Here's how the part is built. I have some questions about the finished solid (model axes, mm). A direction names the side the tool comes from. Give positions to 0.01 mm unless a question says otherwise; leave off trailing zeros. Order: outer loops, then holes, each group sorted by start corner. A loop starts at its lowest first (then second) coordinate and runs counter-clockwise, first axis right, second up.
Autodesk Inventor part; units mm, degrees
ref_plane "YZ Plane" through (0, 0, 0) normal (1, 0, 0) x (0, 1, 0)
ref_plane "XZ Plane" through (0, 0, 0) normal (0, 1, 0) x (-1, 0, 0)
ref_plane "XY Plane" through (0, 0, 0) normal (0, 0, 1) x (1, 0, 0)
sketch "Sketch1" plane through (0, 0, 0) normal (0, 1, 0) x (-1, 0, 0)
  line L0 (90, 60) -> (-90, 60)
  line L1 (-90, 60) -> (-90, -60)
  line L2 (-90, -60) -> (90, -60)
  line L3 (90, -60) -> (90, 60)
  line L4 (90, 60) -> (-90, -60) construction
  line L5 (-90, 60) -> (90, -60) construction
  point P0 (0, 0)
  dimension "d0" = 180
  dimension "d1" = 120
extrude "Extrusion1" add sketch "Sketch1" along normal blind 15
fillet "Face Fillet1" radius 5 1 edges at (90, 7.5, 60)
fillet "Face Fillet2" radius 5 1 edges at (90, 7.5, -60)
fillet "Face Fillet3" radius 5 1 edges at (-90, 7.5, -60)
fillet "Face Fillet4" radius 5 1 edges at (-90, 7.5, 60)
sketch "Sketch2" plane through (0, 15, 0) normal (0, 1, 0) x (1, 0, 0)
  circle A0 centre (0, 0) radius 50
  dimension "d8" = 100
extrude "Extrusion2" add sketch "Sketch2" along normal blind 10
sketch "Sketch3" plane through (0, 25, 0) normal (0, 1, 0) x (1, 0, 0)
  circle A0 centre (0, 0) radius 35
  dimension "d11" = 70
extrude "Extrusion3" add sketch "Sketch3" along normal blind 10
properties part number "base_of weel"
Q1. I need wall thicknesses on L1, parallel to Y at x = 68, z = 5.5; L2, parallel to Y at x = -35, z = 30; L3, parallel to Z at x = 4, y = 29.5. Which ranges of each line are inside material? Lowest first, please.
Filled sheet:
L1: y = 0 to 15
L2: y = 0 to 25
L3: z = -34.77 to 34.77
Q2. If we section it at C-C on y = 31: List the corners of the cut face in (x, z) for me, plus the area to 3 significant figures.
Filled sheet:
outline: circle Ø70 at (0, 0)
area: 3,850 mm2
Q3. If we section it at B-B on z = 0: List the corners of the cut face in (x, y) for me, plus the area to 3 significant figures.
Filled sheet:
outline: (-90, 0) - (90, 0) - (90, 15) - (50, 15) - (50, 25) - (35, 25) - (35, 35) - (-35, 35) - (-35, 25) - (-50, 25) - (-50, 15) - (-90, 15) - close
area: 4,400 mm2
Q4. I'm going to push flat-ended pins straight in: P1, Ø3, axis at x = -54, z = -14, coming from the +Y side; P2, Ø2, axis at y = 24.5, z = 16, coming from the -X side; P3, Ø2, axis at x = 38, z = 14, coming from the +Y side. Where does each tip first touch, or does it pass through?
Filled sheet:
P1: stops at y = 15
P2: stops at x = -47.7
P3: stops at y = 25
Q5. If we section it at A-A on x = 0: List the corners of the cut face in (y, z) for me, plus the area to 3 significant figures.
Filled sheet:
outline: (0, -60) - (15, -60) - (15, -50) - (25, -50) - (25, -35) - (35, -35) - (35, 35) - (25, 35) - (25, 50) - (15, 50) - (15, 60) - (0, 60) - close
area: 3,500 mm2
Q6. If we section it at D-D on x = -65.5: List the corners of the cut face in (y, z) for me.
Filled sheet:
outline: (0, -60) - (15, -60) - (15, 60) - (0, 60) - close
Q7. For faces 1 (the face through (0, 35, 0)), 2 (the face through (-34, 25, 10)), which set-ups out of +Z, -Z, +X, -X, +Y, -Y let a thin tool reach every point of the face, with its end or its side?
Filled sheet:
face 1: +Z, -Z, +X, -X, +Y
face 2: +Y
